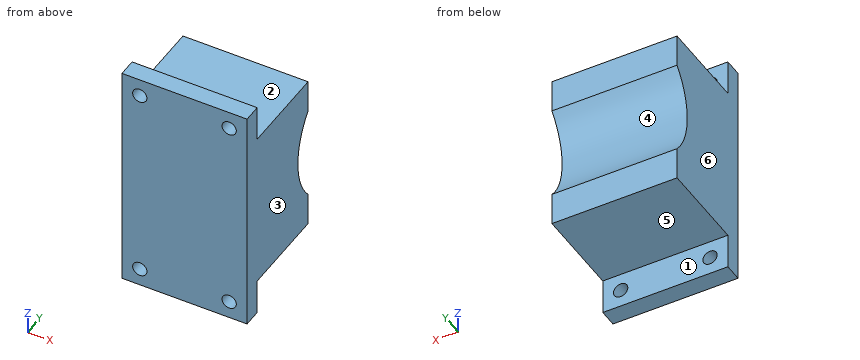
```python
from build123d import *

# Parameters (mm, degrees)
EXTRUDE_1_DEPTH     = 35
SKETCH_5_R          = 2
CUT_EXTRUDE_2_DEPTH = 10


with BuildPart() as part:
    # 草图3 → 凸台-拉伸1 (new body)
    with BuildSketch(Plane(origin=(0, 0, 0), x_dir=(0, 0, -1), z_dir=(1, 0, 0))):
        with BuildLine():
            Line((37.055330611, 5.099345853), (46.308021103, 5.099345853))
            Line((46.308021103, 5.099345853), (46.308021103, -19.900654147))
            Line((46.308021103, -19.900654147), (56.308021103, -19.900654147))
            Line((56.308021103, -19.900654147), (56.308021103, -24.900654147))
            Line((56.308021103, -24.900654147), (-8.691978897, -24.900654147))
            Line((-8.691978897, -24.900654147), (-8.691978897, -19.900654147))
            Line((-8.691978897, -19.900654147), (1.308021103, -19.900654147))
            Line((1.308021103, -19.900654147), (1.308021103, 5.099345853))
            Line((1.308021103, 5.099345853), (10.560711596, 5.099345853))
            ThreePointArc((10.560711596, 5.099345853), (23.808021103, 0.087069391), (37.055330611, 5.099345853))
        make_face()
    extrude(amount=EXTRUDE_1_DEPTH)

    # 草图5 → 切除-拉伸2 (cut)
    with BuildSketch(Plane(origin=(0, -24.900654147, 0), x_dir=(-1, 0, 0), z_dir=(0, -1, 0))):
        with Locations(Location((-30, -3.691978897, 0), (0, 0, 90))):
            Circle(SKETCH_5_R)
        with Locations(Location((-5, -3.691978897, 0), (0, 0, 90))):
            Circle(SKETCH_5_R)
        with Locations(Location((-30, 51.308021103, 0), (0, 0, 90))):
            Circle(SKETCH_5_R)
        with Locations(Location((-5, 51.308021103, 0), (0, 0, 90))):
            Circle(SKETCH_5_R)
    extrude(amount=-CUT_EXTRUDE_2_DEPTH, mode=Mode.SUBTRACT)


solid = part.part
```
The listing builds one solid part. Answer for the finished solid, in the listing's coordinates (mm). Face numbers are marked on the shaded views. A direction names the side the tool comes from. Coordinates: 2 decimals unless noted, no trailing zeros. Loops run counter-clockwise (first coordinate to the right, second up) from the corner with the lowest first, then second, coordinate; pieces in that order, holes last. Notation, with made-up numbers: M -30,-16 L 2,-16 A21 cw 2,20 Z; hole C 22,-36.5 d8. An arc over 180 degrees is marked long. Answer as a JSON object with one key per item and string values. Group by question number.
Item 1: Section A-A (x = 5) is taken. Write down the section's boundary in (y, z).
Item 2: Each of these flat-tipped pins is pushed along its axis until it touches: P1, Ø2.5, axis at x = 5, z = 3.69, coming from the +Y side; P2, Ø8, axis at x = 22.5, z = -52.5, coming from the +Y side; P3, Ø1, axis at x = 29, z = -28, coming from the +Y side; P4, Ø12.5, axis at x = 11, y = -12, coming from the -Z side. Where does it stop, or does it pass through?
Item 3: Section C-C (x = 16) is taken. Write down the section's boundary in (y, z).
Item 4: Which of the six approach directions +Z, -Z, +X, -X, +Y, -Y give full straight-line access (tool end or side, diameter ignored) to the marked faces 1, 2 and 3?
Item 5: Section D-D (z = -25.5) is taken. Write down the section's boundary in (x, y), and give its area (3 significant figures).
Item 6: Determine the mould class of the marked faces 4, 5 and 6 for opening direction Z: +Z half, -Z half, draft (parallel to the pull), parting line (faces both ways), or undercut.
Item 7: Consider L1, parallel to Z at x = 21, y = -6; L2, parallel to Z at x = 14.5, y = 3.5; L3, parallel to Y at x = 22.5, z = 3.5. Determine where each line is inside the solid, lowest interval first.
Item 8: Section B-B (y = 1.75) is taken. Write down the section's boundary in (x, z).
Solved:
{
 "1": {"outline": "M -24.9,-56.31 L -19.9,-56.31 L -19.9,-53.31 L -24.9,-53.31 Z; M -24.9,-49.31 L -19.9,-49.31 L -19.9,-46.31 L 5.1,-46.31 L 5.1,-37.06 A20.01 cw 5.1,-10.56 L 5.1,-1.31 L -19.9,-1.31 L -19.9,1.69 L -24.9,1.69 Z; M -24.9,5.69 L -19.9,5.69 L -19.9,8.69 L -24.9,8.69 Z"},
 "2": {"P1": "passes through", "P2": "stops at y = -19.9", "P3": "stops at y = 0.64", "P4": "stops at z = -46.31"},
 "3": {"outline": "M -24.9,-56.31 L -19.9,-56.31 L -19.9,-46.31 L 5.1,-46.31 L 5.1,-37.06 A20.01 cw 5.1,-10.56 L 5.1,-1.31 L -19.9,-1.31 L -19.9,8.69 L -24.9,8.69 Z"},
 "4": {"face 1": "-Z, +X, -X, +Y", "face 2": "+Z, +X, -X, +Y", "face 3": "+Z, -Z, +X, +Y, -Y"},
 "5": {"outline": "M 0,-24.9 L 35,-24.9 L 35,0.16 L 0,0.16 Z", "area": "877 mm2"},
 "6": {"face 4": "undercut", "face 5": "-Z half", "face 6": "draft"},
 "7": {"L1": "z = -46.31 to -1.31", "L2": "z = -46.31 to -34.99, -12.63 to -1.31", "L3": "y = -24.9 to -19.9"},
 "8": {"outline": "M 0,-46.31 L 35,-46.31 L 35,-31.8 L 0,-31.8 Z; M 0,-15.82 L 35,-15.82 L 35,-1.31 L 0,-1.31 Z"}
}
